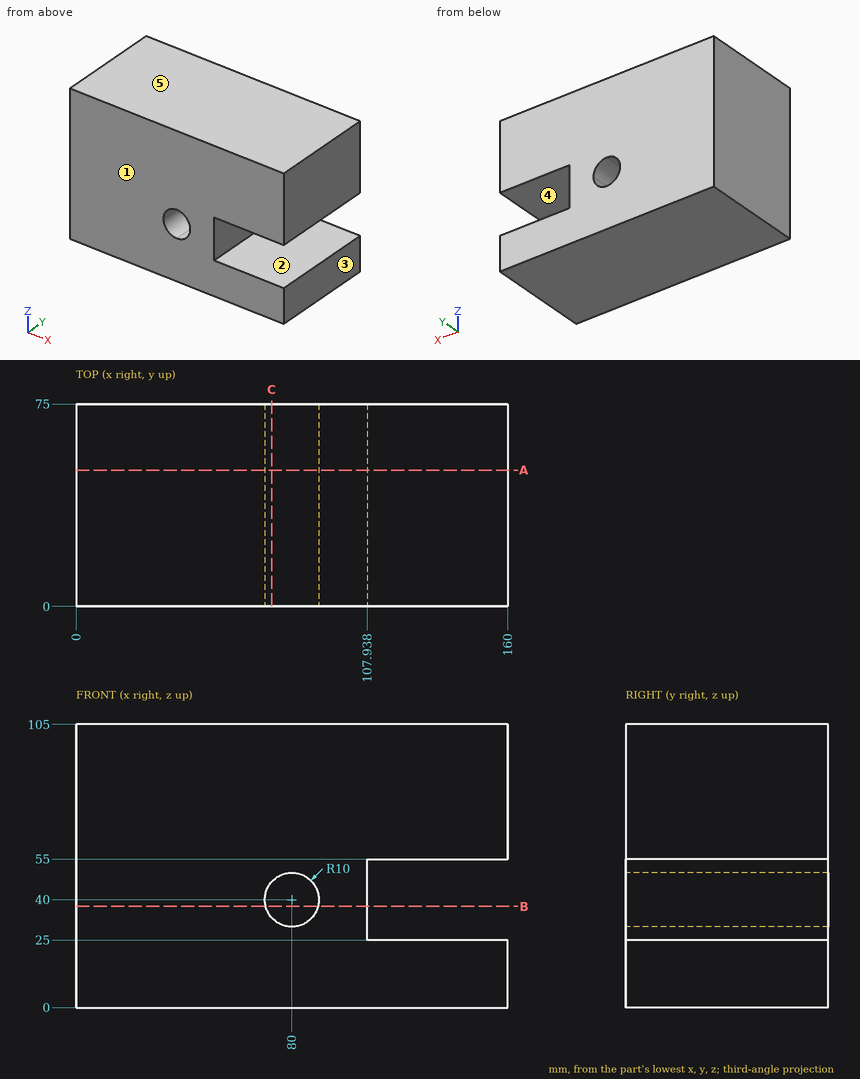
Verification items for this drawing (mm, ordinates from the low corner). A direction names the side the tool comes from. Round coordinates to 2 decimals unless told otherwise and drop trailing zeros. Order: outer loops, then holes, each group sorted by start corner. A loop starts at its lowest first (then second) coordinate and runs counter-clockwise, first axis right, second up. Notation, with made-up numbers: M 24,75.25 L 80,75.25 A20 ccw 80,99.25 Z; hole C 74.25,-9 d6. An arc over 180 degrees is marked long. Answer in a Markdown table with one row per item. Add a question column.
Item 1: Sectioned sample at A-A, the plane y = 50.5. Enter the section's corners in (x, z), plus the area to 3 significant figures.
Item 2: Material ranges on L1, parallel to Z at x = 125, y = 35; L2, parallel to Z at x = 86, y = 12.5; L3, parallel to X at y = 63.5, z = 52, recorded low to high. Write a range as [from, to].
Item 3: Draft check along Z on the marked faces 3, 4 and 5. Enter one of: released by +Z, released by -Z, zero draft, split by the parting line, or undercut.
Item 4: Sectioned sample at B-B, the plane z = 37.5. Enter the section's corners in (x, y).
Item 5: Set-up check for the marked faces 1 and 2: record each of +Z, -Z, +X, -X, +Y, -Y from which the full face is reachable in a straight line by a thin tool's end or side.
Item 6: Sectioned sample at C-C, the plane x = 72.5. Enter the section's corners in (y, z).
Item 7: Depth check by flat-ended pin: pin 1 Ø6 at (y, z) = (12, 50) entering from +X. Enter the tip coordinate at first touch or a pass-through.
Filled in:
| question | item | result |
|---|---|---|
| 1 | outline | M 0,0 L 160,0 L 160,25 L 107.94,25 L 107.94,55 L 160,55 L 160,105 L 0,105 Z; hole C 80,40 d20 |
| 1 | area | 14,900 mm² |
| 2 | L1 | z = [0, 25], [55, 105] |
| 2 | L2 | z = [0, 32], [48, 105] |
| 2 | L3 | x = [0, 107.94] |
| 3 | face 3 | zero draft |
| 3 | face 4 | undercut |
| 3 | face 5 | released by +Z |
| 4 | outline | M 0,0 L 70.32,0 L 70.32,75 L 0,75 Z; M 89.68,0 L 107.94,0 L 107.94,75 L 89.68,75 Z |
| 5 | face 1 | +Z, -Z, +X, -X, -Y |
| 5 | face 2 | +X, +Y, -Y |
| 6 | outline | M 0,0 L 75,0 L 75,33.39 L 0,33.39 Z; M 0,46.61 L 75,46.61 L 75,105 L 0,105 Z |
| 7 | pin 1 | stops at x = 107.94 |
